from build123d import *

# Parameters (mm, degrees)
SKETCH3_R           = 1.5
CUT_EXTRUDE1_DEPTH  = 151.389261732
SKETCH4_R           = 3.5
SKETCH4_R_2         = 1.3
BOSS_EXTRUDE1_DEPTH = 10
SKETCH5_R           = 3.3
SKETCH6_R           = 1.5


# Read off the part's stored shape, not the designer's step: Mirror2, Mirror3
with BuildPart() as part:
    # Sketch1 → Loft1 section 0
    with BuildSketch(Plane(origin=(0, 0, 0), x_dir=(1, 0, 0), z_dir=(0, 1, 0))):
        with BuildLine():
            Line((0, 0), (111.7, 0))
            Line((111.7, 0), (111.7, -100.2))
            Line((111.7, -100.2), (0, -100.2))
            Line((0, -100.2), (0, 0))
        make_face()
    # Sketch2 → Loft1 section 1
    with BuildSketch(Plane(origin=(0, 10, 0), x_dir=(1, 0, 0), z_dir=(0, 1, 0))):
        with BuildLine():
            Line((10, -10), (10, -90.2))
            Line((10, -90.2), (101.7, -90.2))
            Line((101.7, -90.2), (101.7, -10))
            Line((101.7, -10), (10, -10))
        make_face()
    loft()

    # Sketch3 → Cut-Extrude1 (cut, through all)
    with BuildSketch(Plane.XZ):
        with Locations(Location((5, 15, 0), (0, 0, 270))):
            Circle(SKETCH3_R)
        with Locations(Location((5, 85.2, 0), (0, 0, 180))):
            Circle(SKETCH3_R)
        with Locations(Location((106.7, 85.2, 0), (0, 0, 270))):
            Circle(SKETCH3_R)
        with Locations((106.7, 15)):
            Circle(SKETCH3_R)
        with Locations(Location((15, 5, 0), (0, 0, 270))):
            Circle(SKETCH3_R)
        with Locations(Location((15, 95.2, 0), (0, 0, 270))):
            Circle(SKETCH3_R)
        with Locations(Location((96.7, 95.2, 0), (0, 0, 90))):
            Circle(SKETCH3_R)
        with Locations(Location((96.7, 5, 0), (0, 0, 270))):
            Circle(SKETCH3_R)
    extrude(amount=-CUT_EXTRUDE1_DEPTH, mode=Mode.SUBTRACT)

    # Sketch4 → Boss-Extrude1 (add)
    # profile 1 of 4: a face of its own
    with BuildSketch(Plane(origin=(0, 10, 0), x_dir=(1, 0, 0), z_dir=(0, 1, 0))):
        with Locations(Location((81.6, -70.1, 0), (0, 0, 270))):
            Circle(SKETCH4_R)
        with Locations(Location((81.6, -70.1, 0), (0, 0, 270))):
            Circle(SKETCH4_R_2, mode=Mode.SUBTRACT)
    # profile 2 of 4: a face of its own
    with BuildSketch(Plane(origin=(0, 10, 0), x_dir=(1, 0, 0), z_dir=(0, 1, 0))):
        with Locations(Location((81.6, -30.1, 0), (0, 0, 90))):
            Circle(SKETCH4_R)
        with Locations(Location((81.6, -30.1, 0), (0, 0, 90))):
            Circle(SKETCH4_R_2, mode=Mode.SUBTRACT)
    # profile 3 of 4: a face of its own
    with BuildSketch(Plane(origin=(0, 10, 0), x_dir=(1, 0, 0), z_dir=(0, 1, 0))):
        with Locations(Location((41.6, -70.1, 0), (0, 0, 90))):
            Circle(SKETCH4_R)
        with Locations(Location((41.6, -70.1, 0), (0, 0, 90))):
            Circle(SKETCH4_R_2, mode=Mode.SUBTRACT)
    # profile 4 of 4: a face of its own
    with BuildSketch(Plane(origin=(0, 10, 0), x_dir=(1, 0, 0), z_dir=(0, 1, 0))):
        with Locations(Location((41.6, -30.1, 0), (0, 0, 270))):
            Circle(SKETCH4_R)
        with Locations(Location((41.6, -30.1, 0), (0, 0, 270))):
            Circle(SKETCH4_R_2, mode=Mode.SUBTRACT)
    extrude(amount=BOSS_EXTRUDE1_DEPTH)

    # Sketch5 → Cut-Loft1 section 0
    with BuildSketch(Plane.XZ):
        with Locations((106.7, 85.2)):
            Circle(SKETCH5_R)
    # Sketch6 → Cut-Loft1 section 1
    with BuildSketch(Plane(origin=(0, 2.8, 0), x_dir=(-1, 0, 0), z_dir=(0, -1, 0))):
        with Locations((-106.7, -85.2)):
            Circle(SKETCH6_R)
    cut_loft1 = loft(mode=Mode.SUBTRACT)

    # Mirror1: Cut-Loft1 across plane
    add(cut_loft1.mirror(Plane(origin=(5.75, 0, -5.75), x_dir=(0.7071067811865476, 0, 0.7071067811865476), z_dir=(0.7071067811865477, 0, -0.7071067811865475))), mode=Mode.SUBTRACT)

    # Mirror2 outline → Mirror2 (revolve, cut)
    with BuildSketch(Plane(origin=(106.7, 0, 15), x_dir=(1, 0, 0), z_dir=(0, 0, 1))):
        Polygon((3.3, 0), (1.5, 2.8), (1.5, 0), align=None)
    revolve(axis=Axis((106.7, 0, 15), (0, 1, 0)), mode=Mode.SUBTRACT)

    # Mirror2 2 outline → Mirror2 2 (revolve, cut)
    with BuildSketch(Plane(origin=(96.7, 0, 5), x_dir=(1, 0, 0), z_dir=(0, 0, 1))):
        Polygon((3.3, 0), (1.5, 2.8), (1.5, 0), align=None)
    revolve(axis=Axis((96.7, 0, 5), (0, 1, 0)), mode=Mode.SUBTRACT)

    # Mirror3 outline → Mirror3 (revolve, cut)
    with BuildSketch(Plane(origin=(5, 0, 85.2), x_dir=(1, 0, 0), z_dir=(0, 0, 1))):
        Polygon((3.3, 0), (1.5, 2.8), (1.5, 0), align=None)
    revolve(axis=Axis((5, 0, 85.2), (0, 1, 0)), mode=Mode.SUBTRACT)

    # Mirror3 2 outline → Mirror3 2 (revolve, cut)
    with BuildSketch(Plane(origin=(15, 0, 95.2), x_dir=(1, 0, 0), z_dir=(0, 0, 1))):
        Polygon((3.3, 0), (1.5, 2.8), (1.5, 0), align=None)
    revolve(axis=Axis((15, 0, 95.2), (0, 1, 0)), mode=Mode.SUBTRACT)

    # Mirror3 3 outline → Mirror3 3 (revolve, cut)
    with BuildSketch(Plane(origin=(5, 0, 15), x_dir=(1, 0, 0), z_dir=(0, 0, 1))):
        Polygon((3.3, 0), (1.5, 2.8), (1.5, 0), align=None)
    revolve(axis=Axis((5, 0, 15), (0, 1, 0)), mode=Mode.SUBTRACT)

    # Mirror3 4 outline → Mirror3 4 (revolve, cut)
    with BuildSketch(Plane(origin=(15, 0, 5), x_dir=(1, 0, 0), z_dir=(0, 0, 1))):
        Polygon((3.3, 0), (1.5, 2.8), (1.5, 0), align=None)
    revolve(axis=Axis((15, 0, 5), (0, 1, 0)), mode=Mode.SUBTRACT)


solid = part.part
Can you work these out from the model? Positions are in its coordinate system, mm. A direction names the side the tool comes from. Coordinates: 2 decimals unless noted, no trailing zeros. Write each loop counter-clockwise with the first axis right and the second up, starting at its lowest first coordinate (ties: lowest second). Pieces come first, ordered by that corner, then holes. Notation, with made-up numbers: (55.25, 14) -> (97.25, 14) arc R13 cw to (97.25, 28) -> close; hole circle Ø4 at (29.25, 31). An arc over 180 degrees is marked (long way). Write each question's results on one line, items separated by ' | '. Start each with the question number.
Q1. We'd pull the mould along Z, two halves only. Please class faces 3 (the face through (98.351, 2.353, 5.685)), 4 (the face through (81.6, 20, 28.6)), 5 (the face through (108.351, 2.353, 15.685)): +Z half, -Z half, draft (parallel to the pull), parting line (faces both ways), or undercut.
Q2. If I drill on probe 1 along X at (y, z) = (15, 70.1); probe 2 along Z at (x, y) = (5, 3.6); probe 3 along Y at (x, z) = (75, 20.5), over which ranges is the centre line in solid material (lowest first)?
Q3. I'm going to push flat-ended pins straight in: pin 1 (1.3 mm diameter, centred on x = 41.5, z = 30.5, fed in from +Y); pin 2 (2 mm diameter, centred on x = 81.6, z = 30.1, fed in from -Y); pin 3 (1.5 mm diameter, centred on x = 39.5, y = 15, fed in from -Z); pin 4 (1 mm diameter, centred on y = 8.5, z = 14.5, fed in from -X). Where does each tip first touch, or does it pass through?
Q4. Imagine slicing it at B-B (z = 85.2). State how many separate pieces and enclosed holes the cut face has, then the cut area to 3 significant figures.
Q5. On a 3-axis mill with a long thin cutter (end or side, diameter ignored), from which of +Z, -Z, +X, -X, +Y, -Y can I reach the whole of each face in a straight line? I mean faces 1 (the face through (56, 0, 49)), 2 (the face through (82.65, 14.93, 73.44)). Say none if no direction works.
Q6. Imagine slicing it at A-A (y = 13.5). Write out the boundary of the cut face in (x, z).
Taken from the geometry:
1) face 3: undercut | face 4: draft | face 5: undercut
2) probe 1: x = 38.1 to 40.3, 42.9 to 45.1, 78.1 to 80.3, 82.9 to 85.1 | probe 2: z = 3.6 to 13.5, 16.5 to 83.7, 86.7 to 96.6 | probe 3: y = 0 to 10
3) pin 1: stops at y = 10 | pin 2: stops at y = 0 | pin 3: stops at z = 26.87 | pin 4: stops at x = 8
4) separate pieces: 3 | enclosed holes: 0 | area: 977 mm^2
5) face 1: +Z, -Z, +X, -X, -Y | face 2: +Y
6) outline: circle Ø7 at (41.6, 30.1); circle Ø7 at (41.6, 70.1); circle Ø7 at (81.6, 30.1); circle Ø7 at (81.6, 70.1); hole circle Ø2.6 at (41.6, 30.1); hole circle Ø2.6 at (41.6, 70.1); hole circle Ø2.6 at (81.6, 30.1); hole circle Ø2.6 at (81.6, 70.1)
